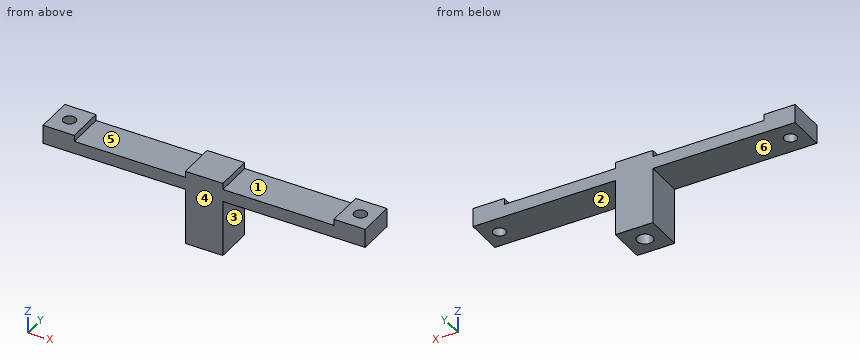
Autodesk Inventor part; units mm, degrees
ref_plane "YZ Plane" through (0, 0, 0) normal (1, 0, 0) x (0, 1, 0)
ref_plane "XZ Plane" through (0, 0, 0) normal (0, 1, 0) x (-1, 0, 0)
ref_plane "XY Plane" through (0, 0, 0) normal (0, 0, 1) x (1, 0, 0)
sketch "Sketch1" plane through (0, 0, 0) normal (0, 0, 1) x (1, 0, 0)
  line L0 (0, 0) -> (51.5, 0)
  line L1 (51.5, 0) -> (51.5, 6)
  line L2 (51.5, 6) -> (0, 6)
  line L3 (0, 6) -> (0, 0)
  dimension "d0" = 6
  dimension "d1" = 51.5
extrude "Extrusion1" add sketch "Sketch1" along normal blind 2
sketch "Sketch2" plane through (0, 0, 2) normal (0, 0, 1) x (1, 0, 0)
  line L0 (0, 0) -> (51.5, 0)
  line L1 (51.5, 0) -> (51.5, 6)
  line L2 (51.5, 6) -> (0, 6)
  line L3 (0, 6) -> (0, 0)
  line L4 (0, 6) -> (5, 6)
  line L5 (5, 6) -> (5, 0)
  line L6 (5, 0) -> (0, 0)
  line L7 (0, 0) -> (0, 6)
  line L8 (22.75, 6) -> (28.75, 6)
  line L9 (28.75, 6) -> (28.75, 0)
  line L10 (28.75, 0) -> (22.75, 0)
  line L11 (22.75, 0) -> (22.75, 6)
  line L12 (51.5, 6) -> (46.5, 6)
  line L13 (46.5, 6) -> (46.5, 0)
  line L14 (46.5, 0) -> (51.5, 0)
  line L15 (51.5, 0) -> (51.5, 6)
  dimension "d4" = 5
  dimension "d5" = 5
  dimension "d7" = 17.75
  dimension "d8" = 17.75
  dimension "d41" = 6
extrude "Extrusion2" add sketch "Sketch2" along normal blind 1 contours L3 L2 L5 L0 | L11 L2 L9 L0 | L13 L2 L1 L0
sketch "Sketch5" plane through (0, 0, 0) normal (0, 0, -1) x (-1, 0, 0)
  line L0 (0, 0) -> (-51.5, 0)
  line L1 (0, 6) -> (0, 0)
  line L2 (-51.5, 6) -> (0, 6)
  line L3 (-51.5, 0) -> (-51.5, 6)
  line L4 (-25.75, 6) -> (-25.75, 0) construction
  line L5 (-51.5, 3) -> (0, 3) construction
  line L6 (-28.75, 6) -> (-22.75, 6)
  line L7 (-22.75, 6) -> (-22.75, 0)
  line L8 (-22.75, 0) -> (-28.75, 0)
  line L9 (-28.75, 0) -> (-28.75, 6)
  line L10 (-28.75, 6) -> (-22.75, 0) construction
  line L11 (-22.75, 6) -> (-28.75, 0) construction
  point P0 (-25.75, 3)
  dimension "d19" = 6
extrude "Extrusion3" add sketch "Sketch5" along normal blind 9 contours L0 L9 L2 L7
sketch "Sketch6" plane through (0, 0, -9) normal (0, 0, -1) x (-1, 0, 0)
  line L0 (-22.75, 0) -> (-22.75, 6)
  line L1 (-22.75, 6) -> (-28.75, 6)
  line L2 (-28.75, 6) -> (-28.75, 0)
  line L3 (-28.75, 0) -> (-22.75, 0)
  line L4 (-28.75, 3) -> (-22.75, 3) construction
  line L5 (-25.75, 6) -> (-25.75, 0) construction
  point P0 (0, 0)
  point P1 (-25.75, 3)
hole "Hole2" at (25.75, 3, -9) direction (0, 0, 1) diameter 2.459 depth 8 tip angle 118
sketch "Sketch7" plane through (0, 0, 0) normal (0, 0, -1) x (-1, 0, 0)
  line L0 (0, 6) -> (0, 0)
  line L1 (0, 0) -> (-22.75, 0)
  line L2 (0, 6) -> (0, 0)
  line L3 (-51.5, 0) -> (-51.5, 6)
  line L4 (-51.5, 6) -> (-28.75, 6)
  line L5 (-51.5, 3) -> (0, 3) construction
  line L6 (-22.75, 6) -> (-22.75, 0)
  line L7 (-28.75, 6) -> (-22.75, 6)
  line L8 (-28.75, 0) -> (-28.75, 6)
  line L9 (-28.75, 0) -> (-51.5, 0)
  line L10 (-22.75, 6) -> (0, 6)
  line L11 (-22.75, 0) -> (-28.75, 0)
  point P0 (-49, 3)
  point P1 (-2.5, 3)
  dimension "d31" = 2.5
  dimension "d32" = 2.5
hole "Hole3" at (49, 3, 0) at (2.5, 3, 0) direction (0, 0, 1) diameter 2.013 depth 3 tip angle 118
properties part number "top_conductor" material "Copper, Alloy"
Read the model definition and answer for the solid it produces. Units are mm, in the model's axes. Face numbers are marked on the shaded views. A direction names the side the tool comes from. Give positions to 0.01 mm unless a question says otherwise; leave off trailing zeros. Write each loop counter-clockwise with the first axis right and the second up, starting at its lowest first coordinate (ties: lowest second). Pieces come first, ordered by that corner, then holes. Notation, with made-up numbers: (79.5, -2.5) -> (127.5, -2.5) arc R15 cw to (127.5, 13.5) -> close; hole circle Ø7 at (81.5, 87.5). An arc over 180 degrees is marked (long way). Answer as a JSON object with one key per item and string values. Group by question number.
1) Find section A-A (x = 2.5). Write down the section's boundary in (y, z).
2) Consider L1, parallel to X at y = 3, z = 2.3; L2, parallel to X at y = 3, z = 0.9; L3, parallel to Y at x = 25.75, z = -6. Determine where each line is inside the solid, lowest interval first. Write a range as from..to.
3) Find section D-D (z = -6.75). Write down the section's boundary in (x, y).
4) The mould has two halves that part along X. Classify the marked faces 1, 2 and 3: +X half, -X half, draft (parallel to the pull), parting line (faces both ways), or undercut.
5) Find section C-C (y = 4.8). Write down the section's boundary in (x, z).
6) A tool of negligible diameter and unlimited length cuts with its end or side. For the marked faces 4, 5 and 6, from which of +Z, -Z, +X, -X, +Y, -Y can it reach the whole face along a straight path? Write none if from no direction.
7) Find section B-B (z = 1.5). Write down the section's boundary in (x, y), and give its area (3 significant figures).
8) Each of these flat-tipped pins is pushed along its axis until it touches: P1, Ø1, axis at y = 0.5, z = -2.5, coming from the +X side; P2, Ø1.5, axis at x = 18, y = 4, coming from the -Z side; P3, Ø3, axis at x = 15, y = 2.5, coming from the +Z side. Where does it stop, or does it pass through?
Values follow:
{
 "1": {"outline": "(0, 0) -> (1.99, 0) -> (1.99, 3) -> (0, 3) -> close; (4.01, 0) -> (6, 0) -> (6, 3) -> (4.01, 3) -> close"},
 "2": {"L1": "x = 0..1.49, 3.51..5, 22.75..28.75, 46.5..47.99, 50.01..51.5", "L2": "x = 0..1.49, 3.51..47.99, 50.01..51.5", "L3": "y = 0..1.77, 4.23..6"},
 "3": {"outline": "(22.75, 0) -> (28.75, 0) -> (28.75, 6) -> (22.75, 6) -> close; hole circle Ø2.46 at (25.75, 3)"},
 "4": {"face 1": "undercut", "face 2": "draft", "face 3": "+X half"},
 "5": {"outline": "(0, 0) -> (22.75, 0) -> (22.75, -9) -> (28.75, -9) -> (28.75, 0) -> (51.5, 0) -> (51.5, 3) -> (46.5, 3) -> (46.5, 2) -> (28.75, 2) -> (28.75, 3) -> (22.75, 3) -> (22.75, 2) -> (5, 2) -> (5, 3) -> (0, 3) -> close"},
 "6": {"face 4": "+Z, -Z, +X, -X, -Y", "face 5": "+Z, +Y, -Y", "face 6": "-Z, -X, +Y, -Y"},
 "7": {"outline": "(0, 0) -> (51.5, 0) -> (51.5, 6) -> (0, 6) -> close; hole circle Ø2.01 at (2.5, 3); hole circle Ø2.01 at (49, 3)", "area": "303 mm2"},
 "8": {"P1": "stops at x = 28.75", "P2": "stops at z = 0", "P3": "stops at z = 2"}
}
